Drawing for the job (mm, zero at the part's lowest x, y, z). A direction names the side the tool comes from. Coordinates: 2 decimals unless noted, no trailing zeros. Write each loop counter-clockwise with the first axis right and the second up, starting at its lowest first coordinate (ties: lowest second). Pieces come first, ordered by that corner, then holes.
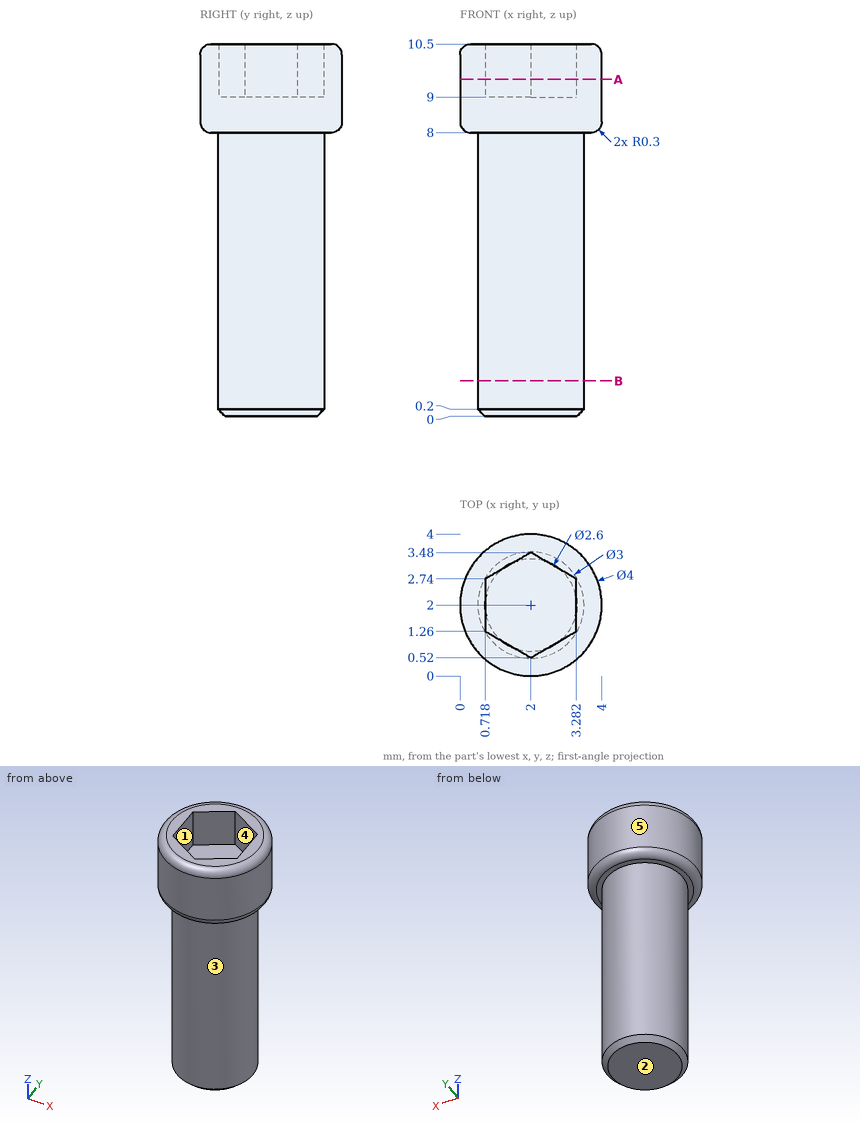
Item 1: Which spindle directions (+Z, -Z, +X, -X, +Y, -Y) get a long thin tool onto all of the face, cutting with end or side? Do the marked faces 4 and 5. Say none if no direction does.
Item 2: Wall check: line 1 along Z through (x, y) = (2.1, 1.65); line 2 along X through (y, z) = (1.75, 0.5); line 3 along Z through (x, y) = (3.65, 2.35). Give the ranges that are in metal, low to high.
Item 3: Two-plate mould, pull along X, no slides. Class the marked faces 1, 2 and 3: +X half, -X half, draft (parallel to the pull), parting line (faces both ways), or undercut.
Item 4: Flat gauge pins, fed straight in: pin 1 Ø0.7 at (y, z) = (1.5, 10) entering from +X; pin 2 Ø2 at (y, z) = (2, 2) entering from -X; pin 3 Ø0.8 at (x, y) = (1.5, 2) entering from +Z. Where does each tip first touch, or does it go through?
Item 5: Saw through at B-B, the plane z = 1. Write the cut outline in (x, y).
Item 6: Saw through at A-A, the plane z = 9.5. Write the cut outline in (x, y).
Working result:
1. face 4: +Z
1. face 5: +Z, -Z
2. line 1: z = 0 to 9
2. line 2: x = 0.52 to 3.48
2. line 3: z = 8 to 10.5
3. face 1: undercut
3. face 2: draft
3. face 3: parting line
4. pin 1: stops at x = 3.99
4. pin 2: stops at x = 0.5
4. pin 3: stops at z = 9
5. outline: circle Ø3 at (2, 2)
6. outline: circle Ø4 at (2, 2); hole (0.72, 1.26) - (2, 0.52) - (3.28, 1.26) - (3.28, 2.74) - (2, 3.48) - (0.72, 2.74) - close
